from build123d import *

# Parameters (mm, degrees)
F0_R     = 9.525
F1_DEPTH = 82.55
F2_R     = 19.05
F3_DEPTH = 3.175
F4_R     = 6.35
F5_DEPTH = 53.975
F6_R     = 5.08
F7_SIZE  = 1.5875
F8_W     = 1.5875
F8_H     = 25.4
F9_DEPTH = 25.4
F10_SIZE = 0.8001


with BuildPart() as f1:
    # F0 (on Top) → F1 (new body)
    with BuildSketch(Plane.XY):
        Circle(F0_R)
    extrude(amount=F1_DEPTH)

    # F2 (on Top) → F3 (join)
    with BuildSketch(Plane.XY):
        Circle(F2_R)
    extrude(amount=F3_DEPTH)

    # F4 (on face) → F5 (cut)
    with BuildSketch(Plane.XY.offset(82.55)):
        Circle(F4_R)
    extrude(amount=-F5_DEPTH, mode=Mode.SUBTRACT)

    # F6
    f6_edges = [f1.edges().sort_by_distance(p)[0] for p in [
        (-9.525, 0, 3.175),
    ]]
    fillet(f6_edges, radius=F6_R)

    # F7
    f7_edges = [f1.edges().sort_by_distance(p)[0] for p in [
        (-9.525, 0, 82.55),
        (-19.05, 0, 3.175),
    ]]
    chamfer(f7_edges, length=F7_SIZE)

    # F8 (on face) → F9 (cut)
    with BuildSketch(Plane.XY.offset(82.55)):
        Polygon((1.5875, 0), (0, 0), (0, 25.4), (-1.5875, 25.4), (-1.5875, 0), (-1.5875, -25.4), (0, -25.4), (1.5875, -25.4), align=None)
        with Locations((0.79375, 12.7)):
            Rectangle(F8_W, F8_H)
    extrude(amount=-F9_DEPTH, mode=Mode.SUBTRACT)

    # F10
    f10_edges = [f1.edges().sort_by_distance(p)[0] for p in [
        (1.5875, 7.770069, 57.15),
        (1.5875, -7.770069, 57.15),
        (-1.5875, 7.770069, 57.15),
        (-1.5875, -7.770069, 57.15),
    ]]
    chamfer(f10_edges, length=F10_SIZE)


solid = f1.part
Can you work these out from the model? Positions are in its coordinate system, mm. A direction names the side the tool comes from. Give positions to 0.01 mm unless a question says otherwise; leave off trailing zeros. Write each loop counter-clockwise with the first axis right and the second up, starting at its lowest first coordinate (ties: lowest second). Pieces come first, ordered by that corner, then holes. Notation, with made-up numbers: (31.25, 14) -> (52.25, 14) arc R14 ccw to (52.25, 30) -> close; hole circle Ø1 at (-26, 84.25). An arc over 180 degrees is marked (long way). Answer as a JSON object with one key per item and string values. Group by question number.
Item 1: Suppose I cut it at C-C (z = 11.5). Please give me the cut outline in (x, y) (3 decimals), plus the area to 3 significant figures.
Item 2: We'd pull the mould along Y, two halves only. Please class faces 4 (the face through (0, 0, 28.575)), 5 (the face through (0, 0, 0)), 6 (the face through (-8.189, 0.161, 82.297)): +Y half, -Y half, draft (parallel to the pull), parting line (faces both ways), or undercut.
Item 3: For faces 1 (the face through (6.057, 1.907, 55.94)), 2 (the face through (1.588, -8, 70)), 3 (the face through (8.189, -0.161, 82.297)), which set-ups out of +Z, -Z, +X, -X, +Y, -Y let a thin tool reach every point of the face, with its end or its side?
Item 4: I'm going to push flat-ended pins straight in: P1, Ø12, axis at x = -14, z = 44.5, coming from the -Y side; P2, Ø2.5, axis at y = 7, z = 64.5, coming from the -X side; P3, Ø1.6, axis at y = -8, z = 70, coming from the +X side; P4, Ø10, axis at x = 13.5, y = 0.5, coming from the -Z side. Where does each tip first touch, or does it pass through?
Item 5: Please list where these lines run through material, in increasing order: line 1 (Y direction, x = 0, z = 52) (3 decimals); line 2 (X direction, y = 5, z = 40.5); line 3 (Z direction, x = 9, y = -11.5) (3 decimals). Write a range as [from, to].
Findings:
{
 "1": {"outline": "circle Ø19.05 at (0, 0)", "area": "285 mm²"},
 "2": {"face 4": "undercut", "face 5": "draft", "face 6": "parting line"},
 "3": {"face 1": "+Z", "face 2": "+Z, +Y, -Y", "face 3": "+Z, +X"},
 "4": {"P1": "stops at y = -5.17", "P2": "stops at x = -7.59", "P3": "stops at x = 6.24", "P4": "stops at z = 0"},
 "5": {"line 1": "y = [-9.525, -6.35], [6.35, 9.525]", "line 2": "x = [-8.11, -3.91], [3.91, 8.11]", "line 3": "z = [0, 3.175]"}
}
